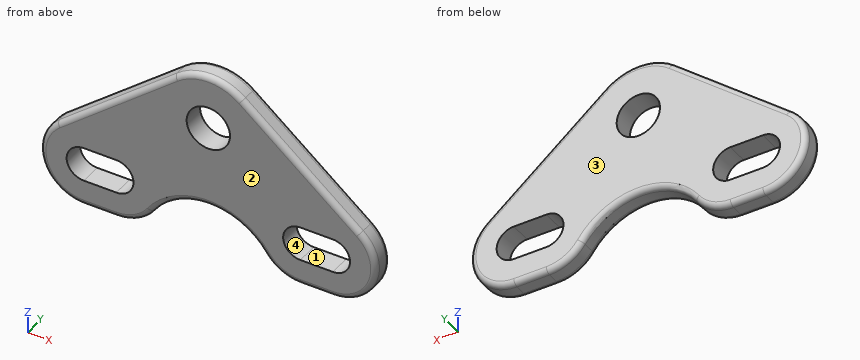
from build123d import *

# Parameters (mm, degrees)
SKETCH1_R           = 4
BOSS_EXTRUDE1_DEPTH = 4
FILLET1_R           = 1


with BuildPart() as part:
    # Sketch1 → Boss-Extrude1 (new body)
    with BuildSketch(Plane(origin=(0, 0, 0), x_dir=(1, 0, 0), z_dir=(0, 1, 0))):
        with BuildLine():
            Line((-28.025651318, -6.22437377), (-6.282064148, -23.780467212))
            ThreePointArc((-6.282064148, -23.780467212), (0, -26), (6.282064148, -23.780467212))
            Line((6.282064148, -23.780467212), (28.025651318, -6.22437377))
            ThreePointArc((28.025651318, -6.22437377), (30.543042826, 2.665052517), (23, 8))
            Line((23, 8), (17, 8))
            ThreePointArc((17, 8), (13.292968107, 7.089281666), (10.429951691, 4.564478636))
            ThreePointArc((10.429951691, 4.564478636), (0, -0.88941153), (-10.429951691, 4.564478636))
            ThreePointArc((-10.429951691, 4.564478636), (-13.292968107, 7.089281666), (-17, 8))
            Line((-17, 8), (-23, 8))
            ThreePointArc((-23, 8), (-30.543042826, 2.665052517), (-28.025651318, -6.22437377))
        make_face()
        with Locations((0, -16)):
            Circle(SKETCH1_R, mode=Mode.SUBTRACT)
        with BuildLine():
            Line((-23, 3.175), (-17, 3.175))
            ThreePointArc((-17, 3.175), (-13.825, 0), (-17, -3.175))
            Line((-17, -3.175), (-23, -3.175))
            ThreePointArc((-23, -3.175), (-26.175, 0), (-23, 3.175))
        make_face(mode=Mode.SUBTRACT)
        with BuildLine():
            Line((17, 3.175), (23, 3.175))
            ThreePointArc((23, 3.175), (26.175, 0), (23, -3.175))
            Line((23, -3.175), (17, -3.175))
            ThreePointArc((17, -3.175), (13.825, 0), (17, 3.175))
        make_face(mode=Mode.SUBTRACT)
    extrude(amount=BOSS_EXTRUDE1_DEPTH)

    # Fillet1
    fillet1_edges = [part.edges().sort_by_distance(p)[0] for p in [
        (0, 4, 26),
        (0, 0, 0.88941153),
        (13.292968107, 0, -7.089281666),
        (20, 0, -8),
        (30.543042826, 0, -2.665052517),
        (17.153857733, 0, 15.002420491),
        (0, 0, 26),
        (-17.153857733, 0, 15.002420491),
        (-30.543042826, 0, -2.665052517),
        (17.153857733, 4, 15.002420491),
        (30.543042826, 4, -2.665052517),
        (20, 4, -8),
        (13.292968107, 4, -7.089281666),
        (0, 4, 0.88941153),
        (-13.292968107, 4, -7.089281666),
        (-20, 4, -8),
        (-30.543042826, 4, -2.665052517),
        (-17.153857733, 4, 15.002420491),
        (-20, 0, -8),
        (-13.292968107, 0, -7.089281666),
    ]]
    fillet(fillet1_edges, radius=FILLET1_R)


solid = part.part
Verification items for the finished model (mm, model axes). Face numbers are marked on the shaded views. A direction names the side the tool comes from. Coordinates: 2 decimals unless noted, no trailing zeros. Loops run counter-clockwise (first coordinate to the right, second up) from the corner with the lowest first, then second, coordinate; pieces in that order, holes last. Notation, with made-up numbers: (45, 12.5) -> (79, 12.5) arc R34 cw to (79, 43.5) -> close; hole circle Ø9 at (74.25, -1.5). An arc over 180 degrees is marked (long way). Answer as a JSON object with one key per item and string values. Group by question number.
Item 1: Scan lines: probe 1 along Z at (x, y) = (25, 1.6); probe 2 along Z at (x, y) = (0, 1.85); probe 3 along X at (y, z) = (3.25, 16). Record each from-to range of solid material in increasing order.
Item 2: Mould release check, pull along X, two halves, no side actions. Record for the marked faces 3 and 4: +X half, -X half, draft (parallel to the pull), parting line (faces both ways), or undercut.
Item 3: Sectioned sample at B-B on y = 2. Record the boundary of the cut face in (x, z) (3 decimals), plus the area to 3 significant figures.
Item 4: Depth check by flat-ended pin: pin 1 (2 mm diameter, centred on x = 15, z = 17, fed in from -Y); pin 2 (4 mm diameter, centred on x = -1, z = -0.5, fed in from -Y); pin 3 (1 mm diameter, centred on y = 1, z = 9.5, fed in from -X). Enter the tip coordinate at first touch or a pass-through.
Item 5: Sectioned sample at A-A on x = 0. Record the boundary of the cut face in (y, z), plus the area to 3 significant figures.
Item 6: Tool access check on the marked faces 1 and 2. Record the directions out of +Z, -Z, +X, -X, +Y, -Y that give a thin tool (end or side, any length) a straight path to the whole face; none if there is none.
Item 7: Sectioned sample at C-C on z = 0. State how many separate pieces and enclosed holes the cut face has, plus the area to 3 significant figures.
Evaluation:
{
 "1": {"probe 1": "z = -7.75 to -2.47, 2.47 to 8.67", "probe 2": "z = 0.89 to 12, 20 to 26", "probe 3": "x = -15.87 to -4, 4 to 15.87"},
 "2": {"face 3": "draft", "face 4": "undercut"},
 "3": {"outline": "(-28.026, 6.224) arc R8 ccw to (-23, -8) -> (-17, -8) arc R8 ccw to (-10.43, -4.564) arc R12.7 cw to (10.43, -4.564) arc R8 ccw to (17, -8) -> (23, -8) arc R8 ccw to (28.026, 6.224) -> (6.282, 23.78) arc R10 ccw to (-6.282, 23.78) -> close; hole (-23, -3.175) -> (-17, -3.175) arc R3.175 ccw to (-17, 3.175) -> (-23, 3.175) arc R3.175 ccw to start; hole circle Ø8 at (0, 16); hole (17, -3.175) -> (23, -3.175) arc R3.175 ccw to (23, 3.175) -> (17, 3.175) arc R3.175 ccw to start", "area": "1,110 mm²"},
 "4": {"pin 1": "stops at y = 0.02", "pin 2": "stops at y = 0.06", "pin 3": "stops at x = -24.59"},
 "5": {"outline": "(0, 1.89) arc R1 ccw to (1, 0.89) -> (3, 0.89) arc R1 ccw to (4, 1.89) -> (4, 12) -> (0, 12) -> close; (0, 20) -> (4, 20) -> (4, 25) arc R1 ccw to (3, 26) -> (1, 26) arc R1 ccw to (0, 25) -> close", "area": "67.6 mm²"},
 "6": {"face 1": "+Y, -Y", "face 2": "+Z, -Z, +X, -X, -Y"},
 "7": {"separate pieces": "4", "enclosed holes": "0", "area": "109 mm²"}
}
